```python
from build123d import *

# Parameters (mm, degrees)
F0_R     = 15.7634364534
F1_DEPTH = 38.1
F2_DEPTH = 38.1
F6_DEPTH = 25.4
F7_DEPTH = 25.4
F8_DEPTH = 25.4


with BuildPart() as f1:
    # F0 (on Front) → F1 (new body)
    with BuildSketch(Plane.XZ):
        Circle(F0_R)
    extrude(amount=F1_DEPTH)

    # F2 (add): a face of the model
    f2_faces = [f1.faces().sort_by_distance(p)[0] for p in [
        (0, 0, 0),
    ]]
    extrude(f2_faces, amount=F2_DEPTH)

    # F5 (on face) → F6 (join)
    with BuildSketch(Plane(origin=(0, 38.1, 0), x_dir=(-1, 0, 0), z_dir=(0, 1, 0))):
        with BuildLine():
            Line((-15.7634364534, 56.6483028233), (-15.7634364534, 0))
            ThreePointArc((-15.7634364534, 0), (0, 15.7634364534), (15.7634364534, 0))
            Line((15.7634364534, 0), (16.0325393081, 0))
            Line((16.0325393081, 0), (16.0325393081, 56.6483028233))
            ThreePointArc((16.0325393081, 56.6483028233), (0.1345514273, 40.7503149426), (-15.7634364534, 56.6483028233))
        make_face()
    extrude(amount=-F6_DEPTH)

    # F3 (on face) → F7 (join)
    with BuildSketch(Plane.XZ.offset(38.1)):
        with BuildLine():
            Line((-15.7634364534, 56.9536834955), (-15.7634364534, 0))
            ThreePointArc((-15.7634364534, 0), (0, 15.7634364534), (15.7634364534, 0))
            Line((15.7634364534, 0), (16.0325393081, 0))
            Line((16.0325393081, 0), (16.0325393081, 56.9536834955))
            Line((16.0325393081, 56.9536834955), (-15.7634364534, 56.9536834955))
        make_face()
    extrude(amount=-F7_DEPTH)

    # F4 (on face) → F8 (join)
    with BuildSketch(Plane.XZ.offset(38.1)):
        with BuildLine():
            Line((-15.7634364534, 56.9536834955), (15.9245655957, 56.9536834955))
            ThreePointArc((15.9245655957, 56.9536834955), (-1.132676387, 72.837915728), (-15.7634364534, 54.6940683534))
            Line((-15.7634364534, 54.6940683534), (-15.7634364534, 56.9536834955))
        make_face()
    extrude(amount=-F8_DEPTH)


solid = f1.part
```
Geometry check sheet. Reference: the model listing, model coordinates, mm. A direction names the side the tool comes from. Round coordinates to 2 decimals unless told otherwise and drop trailing zeros. Loops run counter-clockwise (first coordinate to the right, second up) from the corner with the lowest first, then second, coordinate; pieces in that order, holes last. Notation, with made-up numbers: (10, 14) - (32, 14) arc R22 ccw to (32, 39) - close; hole circle Ø1 at (-38, 0.5). An arc over 180 degrees is marked (long way). Write item = value, one per line. Start each with the question number.
1. Set-up check for faces 5 (the face through (0, 38.1, 13)), 6 (the face through (15.763, 26, 29)): record each of +Z, -Z, +X, -X, +Y, -Y from which the full face is reachable in a straight line by a thin tool's end or side.
2. Section check A-A on z = 39. Enter the section's corners in (x, y).
3. Depth check by flat-ended pin: pin 1 (3 mm diameter, centred on x = -5, y = -27.5, fed in from +Z); pin 2 (2 mm diameter, centred on x = 11.5, y = -12.5, fed in from +Z); pin 3 (5 mm diameter, centred on y = -0.5, z = 17, fed in from +X). Enter the tip coordinate at first touch or a pass-through.
4. Mould release check, pull along X, two halves, no side actions. Record for faces 1 (the face through (-0.484, 25.578, 40.754)), 2 (the face through (-3.42, -0.53, -15.39)), 3 (the face through (16.033, -26, 28)), 4 (the face through (-15.763, -26, 28)): released by +X, released by -X, zero draft, split by the parting line, or undercut.
5. Section check D-D on z = 13.5. Enter the section's corners in (x, y), then the cut area to 3 significant figures.
6. Thickness scan on line 1 (Y direction, x = -1.5, z = 38.5); line 2 (X direction, y = -24, z = 34.5); line 3 (Y direction, x = 1, z = 57). Record the ranges inside material, lowest first.
7. Section check B-B on x = -9. Enter the section's corners in (y, z), then the cut area to 3 significant figures.
8. Section check C-C on y = -24. Enter the section's corners in (x, z), then the cut area to 3 significant figures.
Working result:
q1.face_5 = +Z, -Z, +X, -X, +Y
q1.face_6 = +Z, -Z, +X, +Y
q2.outline = (-16.03, 12.7) - (15.76, 12.7) - (15.76, 38.1) - (-16.03, 38.1) - close; (-15.76, -38.1) - (16.03, -38.1) - (16.03, -12.7) - (-15.76, -12.7) - close
q3.pin_1 = 72.49
q3.pin_2 = 68.91
q3.pin_3 = 6.18
q4.face_1 = undercut
q4.face_2 = split by the parting line
q4.face_3 = released by +X
q4.face_4 = released by -X
q5.outline = (-16.03, 12.7) - (-8.14, 12.7) - (-8.14, -12.7) - (-15.76, -12.7) - (-15.76, -38.1) - (16.03, -38.1) - (16.03, -12.7) - (8.14, -12.7) - (8.14, 12.7) - (15.76, 12.7) - (15.76, 38.1) - (-16.03, 38.1) - close
q5.area = 2,030 mm^2
q6.line_1 = -38.1 to -12.7, 12.7 to 38.1
q6.line_2 = -15.76 to 16.03
q6.line_3 = -38.1 to -12.7
q7.outline = (-38.1, -12.94) - (38.1, -12.94) - (38.1, 43.45) - (12.7, 43.45) - (12.7, 12.94) - (-12.7, 12.94) - (-12.7, 70.09) - (-38.1, 70.09) - close
q7.area = 4,200 mm^2
q8.outline = (-15.76, 0) arc R15.76 ccw to (15.76, 0) - (16.03, 0) - (16.03, 56.95) - (15.92, 56.95) arc R15.92 ccw (long way) to (-15.76, 54.69) - close
q8.area = 2,600 mm^2
